The listing builds one solid part. Answer for the finished solid, in the listing's coordinates (mm). Face numbers are marked on the shaded views. Round coordinates to 2 decimals unless told otherwise and drop trailing zeros. Write each loop counter-clockwise with the first axis right and the second up, starting at its lowest first coordinate (ties: lowest second). Pieces come first, ordered by that corner, then holes. Notation, with made-up numbers: M 50,-37 L 108,-37 A25 ccw 108,-9 Z; hole C 48,68.5 d2. An arc over 180 degrees is marked long. Write each question's results on one line, items separated by ' | '.
from build123d import *

# Parameters (mm, degrees)
F0_R     = 2
F1_DEPTH = 1.6
F2_W     = 8.9
F2_H     = 13
F3_DEPTH = 10.8
F4_W     = 15
F4_H     = 12
F5_DEPTH = 6.1


with BuildPart() as f1:
    # F0 (on Top) → F1 (new body)
    with BuildSketch(Plane.XY):
        with BuildLine():
            Line((-92.75, -21.5), (92.75, -21.5))
            ThreePointArc((92.75, -21.5), (94.164214, -20.914214), (94.75, -19.5))
            Line((94.75, -19.5), (94.75, 19.5))
            ThreePointArc((94.75, 19.5), (94.164214, 20.914214), (92.75, 21.5))
            Line((92.75, 21.5), (-92.75, 21.5))
            ThreePointArc((-92.75, 21.5), (-94.164214, 20.914214), (-94.75, 19.5))
            Line((-94.75, 19.5), (-94.75, -19.5))
            ThreePointArc((-94.75, -19.5), (-94.164214, -20.914214), (-92.75, -21.5))
        make_face()
        with Locations((-91.75, -3.5)):
            Circle(F0_R, mode=Mode.SUBTRACT)
        with Locations((48.75, -3.5)):
            Circle(F0_R, mode=Mode.SUBTRACT)
        with Locations((-91.75, 17.5)):
            Circle(F0_R, mode=Mode.SUBTRACT)
        with Locations((48.75, 17.5)):
            Circle(F0_R, mode=Mode.SUBTRACT)
    extrude(amount=F1_DEPTH)

    # F2 (on face) → F3 (join)
    with BuildSketch(Plane.XY.offset(1.6)):
        with Locations((-80.65, -15)):
            Rectangle(F2_W, F2_H)
    extrude(amount=F3_DEPTH)

    # F4 (on face) → F5 (join)
    with BuildSketch(Plane.XY.offset(1.6)):
        with Locations((-27.75, -17.5)):
            Rectangle(F4_W, F4_H)
    extrude(amount=F5_DEPTH)


solid = f1.part
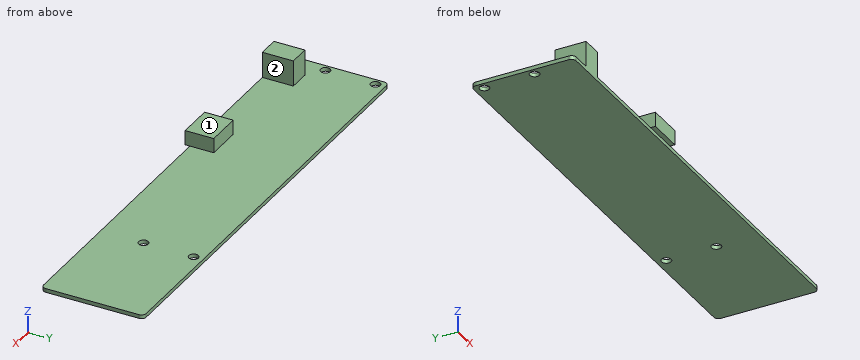
1) Section D-D (y = -16) is taken. Determine the outline of the cut face in (x, z), then the cut area to 3 significant figures.
Return value:
outline: M -94.75,0 L 94.75,0 L 94.75,1.6 L -20.25,1.6 L -20.25,7.7 L -35.25,7.7 L -35.25,1.6 L -76.2,1.6 L -76.2,12.4 L -85.1,12.4 L -85.1,1.6 L -94.75,1.6 Z | area: 491 mm²
2) The mould has two halves that part along X. Classify the marked faces 1 and 2: +X half, -X half, draft (parallel to the pull), parting line (faces both ways), or undercut.
Return value:
face 1: draft | face 2: undercut
3) Section B-B (z = 3.75) is taken. Determine the outline of the cut face in (x, y).
Return value:
outline: M -85.1,-21.5 L -76.2,-21.5 L -76.2,-8.5 L -85.1,-8.5 Z; M -35.25,-23.5 L -20.25,-23.5 L -20.25,-11.5 L -35.25,-11.5 Z
4) Section A-A (y = 17.5) is taken. Determine the outline of the cut face in (x, z).
Return value:
outline: M -94.75,0 L -93.75,0 L -93.75,1.6 L -94.75,1.6 Z; M -89.75,0 L 46.75,0 L 46.75,1.6 L -89.75,1.6 Z; M 50.75,0 L 94.75,0 L 94.75,1.6 L 50.75,1.6 Z
5) Each of these flat-tipped pins is pushed along its axis until it touches: pin 1 (2.5 mm diameter, centred on x = -80, z = 9, fed in from +Y); pin 2 (1.5 mm diameter, centred on x = 73.5, y = 16, fed in from -Z); pin 3 (5.5 mm diameter, centred on y = -14.5, z = 6, fed in from +X); pin 4 (9.5 mm diameter, centred on x = -25, y = -18, fed in from +Z). Where does it stop, or does it pass through?
Return value:
pin 1: y = -8.5 | pin 2: z = 0 | pin 3: x = -20.25 | pin 4: z = 7.7
6) Find the intervals of material crossed by line 1 (Y direction, x = -91.75, z = 0.6); line 2 (X direction, y = -16, z = 2.5); line 3 (Z direction, x = 11, y = 2.5), in increasing order.
Return value:
line 1: -21.5 to -5.5, -1.5 to 15.5, 19.5 to 21.5 | line 2: -85.1 to -76.2, -35.25 to -20.25 | line 3: 0 to 1.6
7) Section C-C (x = 48.75) is taken. Determine the outline of the cut face in (y, z).
Return value:
outline: M -21.5,0 L -5.5,0 L -5.5,1.6 L -21.5,1.6 Z; M -1.5,0 L 15.5,0 L 15.5,1.6 L -1.5,1.6 Z; M 19.5,0 L 21.5,0 L 21.5,1.6 L 19.5,1.6 Z
